Geometry check sheet. Reference: the model listing, model coordinates, mm. A direction names the side the tool comes from. Coordinates: 2 decimals unless noted, no trailing zeros. Write each loop counter-clockwise with the first axis right and the second up, starting at its lowest first coordinate (ties: lowest second). Pieces come first, ordered by that corner, then holes. Notation, with made-up numbers: (-32, 40) -> (7, 40) arc R15 cw to (7, 62) -> close; hole circle Ø11 at (64.25, 28.25). An arc over 180 degrees is marked (long way). Use a Markdown table: item, result.
```python
from build123d import *

# Parameters (mm, degrees)
SKETCH1_W           = 38.1
SKETCH1_H           = 19.05
BOSS_EXTRUDE1_DEPTH = 12.7
SKETCH2_W           = 15.875
SKETCH2_H           = 4.572
BOSS_EXTRUDE2_DEPTH = 25.4
SKETCH2_3_W         = 8.128
SKETCH2_3_H         = 8.128
BOSS_EXTRUDE3_DEPTH = 10.16
FILLET1_R           = 1.905
SKETCH3_R           = 0.635
CUT_EXTRUDE1_DEPTH  = 47.6627796
FILLET2_R           = 3.81
BOSS_EXTRUDE4_START = 6.35
SKETCH4_R           = 5.08
SKETCH4_R_2         = 0.635
BOSS_EXTRUDE4_DEPTH = 6.35
FILLET3_R           = 1.27


with BuildPart() as part:
    # Sketch1 → Boss-Extrude1 (new body)
    with BuildSketch(Plane(origin=(0, 0, 0), x_dir=(1, 0, 0), z_dir=(0, 1, 0))):
        Rectangle(SKETCH1_W, SKETCH1_H)
    extrude(amount=BOSS_EXTRUDE1_DEPTH)

    # Sketch2 → Boss-Extrude2 (add)
    with BuildSketch(Plane(origin=(0, 12.7, 0), x_dir=(1, 0, 0), z_dir=(0, 1, 0))):
        with Locations((0, 7.239)):
            Rectangle(SKETCH2_W, SKETCH2_H)
        Polygon((-7.9375, 4.953), (-7.9375, 9.525), (-19.05, 9.525), (-19.05, -9.525), (-7.9375, -9.525), (-7.9375, -4.953), align=None)
        Polygon((19.05, 9.525), (7.9375, 9.525), (7.9375, 4.953), (7.9375, -4.953), (7.9375, -9.525), (19.05, -9.525), align=None)
        with Locations((0, -7.239)):
            Rectangle(SKETCH2_W, SKETCH2_H)
    extrude(amount=BOSS_EXTRUDE2_DEPTH)

    # Sketch2_3 → Boss-Extrude3 (add)
    with BuildSketch(Plane(origin=(0, 12.7, 0), x_dir=(1, 0, 0), z_dir=(0, 1, 0))):
        Rectangle(SKETCH2_3_W, SKETCH2_3_H)
    extrude(amount=BOSS_EXTRUDE3_DEPTH)

    # Fillet1
    fillet1_edges = [part.edges().sort_by_distance(p)[0] for p in [
        (-4.064, 17.78, 4.064),
        (4.064, 17.78, 4.064),
        (4.064, 17.78, -4.064),
        (-4.064, 17.78, -4.064),
    ]]
    fillet(fillet1_edges, radius=FILLET1_R)

    # Sketch3 → Cut-Extrude1 (cut, through all)
    with BuildSketch(Plane(origin=(0, 0, -9.525), x_dir=(-1, 0, 0), z_dir=(0, 0, -1))):
        with Locations((0, 14.351)):
            Circle(SKETCH3_R)
    extrude(amount=-CUT_EXTRUDE1_DEPTH, mode=Mode.SUBTRACT)

    # Fillet2
    fillet2_edges = [part.edges().sort_by_distance(p)[0] for p in [
        (7.9375, 25.4, 4.953),
        (-7.9375, 25.4, 4.953),
        (-7.9375, 25.4, -4.953),
        (7.9375, 25.4, -4.953),
    ]]
    fillet(fillet2_edges, radius=FILLET2_R)

    # Sketch4 → Boss-Extrude4 (add)
    # profile 1 of 2: a face of its own
    with BuildSketch(Plane(origin=(0, 0, -9.525), x_dir=(-1, 0, 0), z_dir=(0, 0, -1)).offset(BOSS_EXTRUDE4_START)):
        with Locations((0, 14.351)):
            Circle(SKETCH4_R)
        with Locations((0, 14.351)):
            Circle(SKETCH4_R_2, mode=Mode.SUBTRACT)
    # profile 2 of 2: a face of its own
    with BuildSketch(Plane(origin=(0, 0, -9.525), x_dir=(-1, 0, 0), z_dir=(0, 0, -1)).offset(BOSS_EXTRUDE4_START)):
        with BuildLine():
            ThreePointArc((5.08, 14.351), (0, 9.271), (-5.08, 14.351))
            Line((-5.08, 14.351), (-5.08, 0))
            Line((-5.08, 0), (5.08, 0))
            Line((5.08, 0), (5.08, 14.351))
        make_face()
    extrude(amount=-BOSS_EXTRUDE4_DEPTH)

    # Fillet3
    fillet3_edges = [part.edges().sort_by_distance(p)[0] for p in [
        (-6.821576836, 38.1, -3.837076836),
        (-12.065, 0, -9.525),
        (0, 19.431, -9.525),
        (5.08, 7.1755, -9.525),
        (5.08, 0, -12.7),
        (-5.08, 7.1755, -15.875),
        (-5.08, 0, -12.7),
        (0, 19.431, -15.875),
        (5.08, 7.1755, -15.875),
        (0, 0, -15.875),
        (-5.08, 7.1755, -9.525),
        (-19.05, 38.1, 0),
        (0, 38.1, 9.525),
        (19.05, 38.1, 0),
        (0, 38.1, -9.525),
        (0, 0, 9.525),
        (0, 22.86, 4.064),
        (-4.064, 22.86, 0),
        (-19.05, 0, 0),
        (4.064, 22.86, 0),
        (0, 22.86, -4.064),
        (-3.506038418, 22.86, -3.506038418),
        (3.506038418, 22.86, -3.506038418),
        (3.506038418, 22.86, 3.506038418),
        (-3.506038418, 22.86, 3.506038418),
        (12.065, 0, -9.525),
        (19.05, 0, 0),
        (19.05, 19.05, 9.525),
        (-19.05, 19.05, 9.525),
        (-19.05, 19.05, -9.525),
        (19.05, 19.05, -9.525),
        (0, 38.1, 4.953),
        (7.9375, 38.1, 0),
        (0, 38.1, -4.953),
        (-7.9375, 38.1, 0),
        (6.821576836, 38.1, 3.837076836),
        (6.821576836, 38.1, -3.837076836),
        (-6.821576836, 38.1, 3.837076836),
    ]]
    fillet(fillet3_edges, radius=FILLET3_R)


solid = part.part
```
Item 1: Depth check by flat-ended pin: P1, Ø1.1, axis at y = 6.5, z = -12, coming from the -X side; P2, Ø10, axis at y = 21, z = -9.5, coming from the -X side; P3, Ø4, axis at x = 1.5, y = 21, coming from the -Z side; P4, Ø1.7, axis at x = 0.5, z = -1.5, coming from the +Y side. Enter the tip coordinate at first touch or a pass-through.
Answer block:
| item | result |
|---|---|
| P1 | stops at x = -5.08 |
| P2 | stops at x = -19.05 |
| P3 | stops at z = -15.38 |
| P4 | stops at y = 22.86 |
Item 2: Thickness scan on L1, parallel to Z at x = -0.5, y = 35 (3 decimals); L2, parallel to X at y = 36, z = -0.75; L3, parallel to Y at x = 0, z = 2. Record the ranges inside material, lowest first. Write a range as [from, to].
Answer block:
| item | result |
|---|---|
| L1 | z = [-9.525, -4.953], [4.953, 9.525] |
| L2 | x = [-19.05, -7.94], [7.94, 19.05] |
| L3 | y = [0, 13.72], [14.99, 22.86] |
Item 3: Tool access check on faces 1 (the cylindrical face through (-4.718, 0.382, -12.673)), 2 (the cylindrical face through (-18.688, 37.718, 0.116)), 3 (the cylindrical face through (-3.49, 17.21, -3.52)). Record the directions out of +Z, -Z, +X, -X, +Y, -Y that give a thin tool (end or side, any length) a straight path to the whole face; none if there is none.
Answer block:
| item | result |
|---|---|
| face 1 | -Z, -X, -Y |
| face 2 | +Z, -Z, -X, +Y |
| face 3 | +Y |
Item 4: Mould release check, pull along X, two halves, no side actions. Record for faces 4 (the cylindrical face through (18.668, 0.362, -0.116)), 5 (the flat face through (-19.05, 19, 0)), 6 (the cylindrical face through (6.85, 24.93, 3.81)), 7 (the cylindrical face through (12.15, 0.36, -9.14)): +X half, -X half, draft (parallel to the pull), parting line (faces both ways), or undercut.
Answer block:
| item | result |
|---|---|
| face 4 | +X half |
| face 5 | -X half |
| face 6 | undercut |
| face 7 | draft |
Item 5: Section check C-C on z = -12.5. Record the boundary of the cut face in (x, y) (3 decimals), then the cut area to 3 significant figures.
Answer block:
| item | result |
|---|---|
| outline | (-5.08, 1.27) arc R1.27 ccw to (-3.81, 0) -> (3.81, 0) arc R1.27 ccw to (5.08, 1.27) -> (5.08, 14.351) arc R5.08 ccw to (-5.08, 14.351) -> close; hole circle Ø1.27 at (0, 14.351) |
| area | 184 mm^2 |
Item 6: Section check B-B on x = -13. Record the boundary of the cut face in (y, z) (3 decimals), then the cut area to 3 significant figures.
Answer block:
| item | result |
|---|---|
| outline | (0, -8.255) arc R1.27 ccw to (1.27, -9.525) -> (36.83, -9.525) arc R1.27 ccw to (38.1, -8.255) -> (38.1, 8.255) arc R1.27 ccw to (36.83, 9.525) -> (1.27, 9.525) arc R1.27 ccw to (0, 8.255) -> close |
| area | 724 mm^2 |
Item 7: Section check D-D on y = 10. Record the boundary of the cut face in (x, z) (3 decimals).
Answer block:
| item | result |
|---|---|
| outline | (-19.05, -8.255) arc R1.27 ccw to (-17.78, -9.525) -> (-6.35, -9.525) arc R1.27 cw to (-5.08, -10.795) -> (-5.08, -14.605) arc R1.27 ccw to (-3.81, -15.875) -> (3.81, -15.875) arc R1.27 ccw to (5.08, -14.605) -> (5.08, -10.795) arc R1.27 cw to (6.35, -9.525) -> (17.78, -9.525) arc R1.27 ccw to (19.05, -8.255) -> (19.05, 8.255) arc R1.27 ccw to (17.78, 9.525) -> (-17.78, 9.525) arc R1.27 ccw to (-19.05, 8.255) -> close |
